from build123d import *

# Parameters (mm, degrees)
SKETCH1_W           = 60
SKETCH1_H           = 70
BOSS_EXTRUDE1_DEPTH = 10
SKETCH2_W           = 60
SKETCH2_H           = 70
SKETCH2_W_2         = 54
SKETCH2_H_2         = 64
BOSS_EXTRUDE2_DEPTH = 15
SKETCH3_R           = 1.5
BOSS_EXTRUDE3_DEPTH = 5
SKETCH8_R           = 3
SKETCH8_R_2         = 0.4
BOSS_EXTRUDE4_DEPTH = 3
CUT_EXTRUDE1_START  = -4
SKETCH11_R          = 0.4
CUT_EXTRUDE1_DEPTH  = 4
SKETCH12_W          = 21.5
SKETCH12_H          = 5
CUT_EXTRUDE2_DEPTH  = 5
FILLET2_R           = 1
SKETCH18_R          = 1.25
CUT_EXTRUDE6_DEPTH  = 7
SKETCH20_W          = 14.5
SKETCH20_H          = 7.5
CUT_EXTRUDE7_DEPTH  = 7
FILLET3_R           = 2


with BuildPart() as part:
    # Sketch1 → Boss-Extrude1 (new body)
    with BuildSketch(Plane(origin=(0, 0, 0), x_dir=(1, 0, 0), z_dir=(0, 1, 0))):
        with Locations((4.122137405, -1.297709924)):
            Rectangle(SKETCH1_W, SKETCH1_H)
    extrude(amount=BOSS_EXTRUDE1_DEPTH)

    # Sketch2 → Boss-Extrude2 (add)
    with BuildSketch(Plane(origin=(0, 10, 0), x_dir=(1, 0, 0), z_dir=(0, 1, 0))):
        with Locations((4.122137405, -1.297709924)):
            Rectangle(SKETCH2_W, SKETCH2_H)
        with Locations((4.122137405, -1.297709924)):
            Rectangle(SKETCH2_W_2, SKETCH2_H_2, mode=Mode.SUBTRACT)
    extrude(amount=BOSS_EXTRUDE2_DEPTH)

    # Sketch3 → Boss-Extrude3 (add)
    with BuildSketch(Plane(origin=(0, 25, 0), x_dir=(1, 0, 0), z_dir=(0, 1, 0))):
        with Locations(Location((-23.377862595, 31.202290076, 0), (0, 0, 340.528779366))):
            Circle(SKETCH3_R)
        with Locations(Location((31.622137405, 31.202290076, 0), (0, 0, 199.471220634))):
            Circle(SKETCH3_R)
        with Locations(Location((31.622137405, -33.797709924, 0), (0, 0, 109.471220634))):
            Circle(SKETCH3_R)
        with Locations(Location((-23.377862595, -33.797709924, 0), (0, 0, 70.528779366))):
            Circle(SKETCH3_R)
    extrude(amount=BOSS_EXTRUDE3_DEPTH)

    # Sketch8 → Boss-Extrude4 (add)
    # profile 1 of 3: a face of its own
    with BuildSketch(Plane(origin=(0, 10, 0), x_dir=(1, 0, 0), z_dir=(0, 1, 0))):
        with Locations(Location((21.622137405, -19.297709924, 0), (0, 0, 270))):
            Circle(SKETCH8_R)
        with Locations(Location((21.622137405, -19.297709924, 0), (0, 0, 270))):
            Circle(SKETCH8_R_2, mode=Mode.SUBTRACT)
    # profile 2 of 3: a face of its own
    with BuildSketch(Plane(origin=(0, 10, 0), x_dir=(1, 0, 0), z_dir=(0, 1, 0))):
        with Locations(Location((-13.377862595, -19.297709924, 0), (0, 0, 270))):
            Circle(SKETCH8_R)
        with Locations(Location((-13.377862595, -19.297709924, 0), (0, 0, 270))):
            Circle(SKETCH8_R_2, mode=Mode.SUBTRACT)
    # profile 3 of 3: a face of its own
    with BuildSketch(Plane(origin=(0, 10, 0), x_dir=(1, 0, 0), z_dir=(0, 1, 0))):
        with Locations(Location((23.622137405, 25.702290076, 0), (0, 0, 270))):
            Circle(SKETCH8_R)
        with Locations(Location((23.622137405, 25.702290076, 0), (0, 0, 270))):
            Circle(SKETCH8_R_2, mode=Mode.SUBTRACT)
    extrude(amount=BOSS_EXTRUDE4_DEPTH)

    # Sketch11 → Cut-Extrude1 (cut)
    with BuildSketch(Plane(origin=(0, 10, 0), x_dir=(1, 0, 0), z_dir=(0, 1, 0)).offset(CUT_EXTRUDE1_START)):
        with Locations(Location((-13.377862595, -19.297709924, 0), (0, 0, 270))):
            Circle(SKETCH11_R)
        with Locations(Location((21.622137405, -19.297709924, 0), (0, 0, 270))):
            Circle(SKETCH11_R)
        with Locations(Location((23.622137405, 25.702290076, 0), (0, 0, 270))):
            Circle(SKETCH11_R)
    extrude(amount=CUT_EXTRUDE1_DEPTH, mode=Mode.SUBTRACT)

    # Sketch12 → Cut-Extrude2 (cut)
    with BuildSketch(Plane(origin=(0, 0, -33.702290076), x_dir=(-1, 0, 0), z_dir=(0, 0, -1))):
        with Locations((3.627862595, 15.5)):
            Rectangle(SKETCH12_W, SKETCH12_H)
    extrude(amount=-CUT_EXTRUDE2_DEPTH, mode=Mode.SUBTRACT)

    # Fillet2
    fillet2_edges = [part.edges().sort_by_distance(p)[0] for p in [
        (-24.792076158, 30, -31.702290076),
        (33.036350967, 30, -31.702290076),
        (32.122137405, 30, 35.211923486),
        (-23.877862595, 30, 35.211923486),
    ]]
    fillet(fillet2_edges, radius=FILLET2_R)

    # Sketch18 → Cut-Extrude6 (cut)
    with BuildSketch(Plane.XZ):
        with Locations(Location((4.122137405, 23.797709924, 0), (0, 0, 270))):
            Circle(SKETCH18_R)
        with Locations(Location((4.122137405, 1.297709924, 0), (0, 0, 270))):
            Circle(SKETCH18_R)
        with Locations(Location((4.122137405, -21.202290076, 0), (0, 0, 270))):
            Circle(SKETCH18_R)
    extrude(amount=-CUT_EXTRUDE6_DEPTH, mode=Mode.SUBTRACT)

    # Sketch20 → Cut-Extrude7 (cut)
    with BuildSketch(Plane.ZY.offset(25.877862595)):
        with Locations((11.047709924, 16.75)):
            Rectangle(SKETCH20_W, SKETCH20_H)
    extrude(amount=-CUT_EXTRUDE7_DEPTH, mode=Mode.SUBTRACT)

    # Fillet3
    # the kernel refuses this fillet: 2 mm, written as the material it adds along each edge
    with BuildSketch(Plane(origin=(-22.877862595, 5, -30.702290076), x_dir=(0, 0, 1), z_dir=(0, 1, 0)), Plane(origin=(31.122137405, 5, -30.702290076), x_dir=(-1, 0, 0), z_dir=(0, 1, 0))) as fillet3_piece_1:
        with BuildLine():
            CenterArc((FILLET3_R, FILLET3_R), FILLET3_R, 180, 90)
            Line((0, FILLET3_R), (0, 0))
            Line((0, 0), (FILLET3_R, 0))
        make_face()
    extrude(amount=20)
    with BuildSketch(Plane(origin=(-22.877862595, 5, 33.297709924), x_dir=(0, 0, -1), z_dir=(0, 1, 0)), Plane(origin=(31.122137405, 5, 33.297709924), x_dir=(-1, 0, 0), z_dir=(0, 1, 0))) as fillet3_piece_2:
        with BuildLine():
            CenterArc((FILLET3_R, -FILLET3_R), FILLET3_R, 90, 90)
            Line((0, -FILLET3_R), (0, 0))
            Line((0, 0), (FILLET3_R, 0))
        make_face()
    extrude(amount=20)


solid = part.part
Design review of the part built by this model. Coordinates are the model's own, in mm. A direction names the side the tool comes from. Give positions to 0.01 mm unless a question says otherwise; leave off trailing zeros. Order: outer loops, then holes, each group sorted by start corner. A loop starts at its lowest first (then second) coordinate and runs counter-clockwise, first axis right, second up.
1. Add section B-B, the plane z = 6.5. State the section outline as (x, y) points.
Solution:
outline: (-25.88, 0) - (34.12, 0) - (34.12, 25) - (31.12, 25) - (31.12, 10) - (-22.88, 10) - (-22.88, 13) - (-25.88, 13) - close; (-25.88, 20.5) - (-22.88, 20.5) - (-22.88, 25) - (-25.88, 25) - close
2. To check wall thickness, follow L1, parallel to X at y = 16, z = -27.5; L2, parallel to Z at x = 13.5, y = 13.5; L3, parallel to Z at x = 23, y = 11.25. State the ranges of each line that lie inside material, in increasing order.
Solution:
L1: x = -25.88 to -22.88, 31.12 to 34.12
L2: z = -33.7 to -30.7, 33.3 to 36.3
L3: z = -33.7 to -30.7, -28.64 to -22.77, 16.63 to 21.96, 33.3 to 36.3
3. Tool access review of faces 1 (the flat face through (-3, 13, -32)), 2 (the cylindrical face through (4.498, 3.451, 22.605)), 3 (the flat face through (-24, 17, 3.798)), 4 (the flat face through (-25, 25, 1)): name each direction out of +Z, -Z, +X, -X, +Y, -Y from which nothing blocks a thin tool from reaching the whole face with its end or side.
Solution:
face 1: -Z
face 2: -Y
face 3: -X
face 4: +Y
4. Mouldability with a two-part tool opening along X and no side actions: class faces 5 (the cylindrical face through (19.797, 11.479, 16.917)), 6 (the flat face through (-3, 0, 1)) as +X half, -X half, draft (parallel to the pull), parting line (faces both ways), or undercut.
Solution:
face 5: undercut
face 6: draft
5. For pin 1 Ø2.5 at (x, z) = (-24.5, 14) entering from +Y; pin 2 Ø0.8 at (x, z) = (4, 23.5) entering from -Y; pin 3 Ø5 at (x, z) = (22.5, -26) entering from +Y, all flat-tipped, find the tip position at first contact; note any pin that passes through.
Solution:
pin 1: stops at y = 25
pin 2: stops at y = 7
pin 3: stops at y = 13
6. Add section D-D, the plane x = 16. State the section outline as (y, z) points, then the cut area to 3 significant figures.
Solution:
outline: (0, -33.7) - (25, -33.7) - (25, -30.7) - (10, -30.7) - (10, 33.3) - (25, 33.3) - (25, 36.3) - (0, 36.3) - close
area: 790 mm2
7. Add section A-A, the plane x = -3. State the section outline as (y, z) points.
Solution:
outline: (0, -33.7) - (13, -33.7) - (13, -30.7) - (10, -30.7) - (10, 33.3) - (25, 33.3) - (25, 36.3) - (0, 36.3) - close; (18, -33.7) - (25, -33.7) - (25, -30.7) - (18, -30.7) - close
8. Add section C-C, the plane y = 21.75. State the section outline as (x, z) points, then the cut area to 3 significant figures.
Solution:
outline: (-25.88, -33.7) - (34.12, -33.7) - (34.12, 36.3) - (-25.88, 36.3) - close; hole (-22.88, -28.7) arc R2 ccw to (-20.88, -30.7) - (29.12, -30.7) arc R2 ccw to (31.12, -28.7) - (31.12, 31.3) arc R2 ccw to (29.12, 33.3) - (-20.88, 33.3) arc R2 ccw to (-22.88, 31.3) - close
area: 747 mm2
